Part model, mm, in its own coordinate system. A direction names the side the tool comes from. Round coordinates to 2 decimals unless told otherwise and drop trailing zeros. Order: outer loops, then holes, each group sorted by start corner. A loop starts at its lowest first (then second) coordinate and runs counter-clockwise, first axis right, second up. Notation, with made-up numbers: (34, -3) - (92, -3) arc R23 ccw to (92, 21) - close; hole circle Ø7 at (-28, 3). An arc over 180 degrees is marked (long way). Return JSON: item names as keys, results as strings. Group by question number.
Item 1: Saw through at A-A on y = 46.5. List the corners of the cut face in (x, z).
Item 2: Saw through at B-B on z = -22.5. List the corners of the cut face in (x, y).
Item 3: Tool access for faces 1 (the face through (1, 83, -68.5)), 2 (the face through (1, 81, -17)), 3 (the face through (2, 9, -24.5)): list every direction of +Z, -Z, +X, -X, +Y, -Y with a clear straight run to the whole face (end or side of a thin tool).
Item 4: Probe probe 1 along Z at (x, y) = (2.8, 35.5); probe 2 along Y at (x, z) = (1.6, -96.5); probe 3 along Z at (x, y) = (2.15, 7). List the from-to ranges inside material, lowest first.
Item 5: Saw through at D-D on x = 0.5. State how many separate pieces and enclosed holes the cut face has, and give its area (3 significant figures).
Item 6: Drop a flat-ended pin along its axis: pin 1 (2.5 mm diameter, centred on y = 6, z = -8.5, fed in from -X) (3 decimals). Give the stop position or say it passes through.
Item 7: Two-plate mould, pull along Z, no slides. Class faces 4 (the face through (1, 81, -88)), 5 (the face through (1, 40, -105)), 6 (the face through (2, 9, -80.5)): released by +Z, released by -Z, zero draft, split by the parting line, or undercut.
Item 8: Saw through at C-C on y = 6. List the corners of the cut face in (x, z), and give its area (3 significant figures).
```python
from build123d import *

# Parameters (mm, degrees)
CROQUIS1_R              = 1.5
CROQUIS1_W              = 3
CROQUIS1_H              = 32
SALIENTE_EXTRUIR1_DEPTH = 3
CORTAR_EXTRUIR1_DEPTH   = 3
CORTAR_EXTRUIR2_DEPTH   = 3


with BuildPart() as part:
    # Croquis1 → Saliente-Extruir1 (new body)
    with BuildSketch(Plane(origin=(0, 0, 0), x_dir=(0, 0, -1), z_dir=(1, 0, 0))):
        Polygon((0, 0), (105, 0), (105, 81), (84.5, 81), (84.5, 84), (68.5, 84), (68.5, 81), (36.5, 81), (36.5, 84), (20.5, 84), (20.5, 81), (0, 81), align=None)
        with Locations((8.5, 71)):
            Circle(CROQUIS1_R, mode=Mode.SUBTRACT)
        with Locations((96.5, 71)):
            Circle(CROQUIS1_R, mode=Mode.SUBTRACT)
        with Locations((8.5, 6)):
            Circle(CROQUIS1_R, mode=Mode.SUBTRACT)
        with Locations(Location((96.5, 6, 0), (0, 0, 180))):
            Circle(CROQUIS1_R, mode=Mode.SUBTRACT)
        with Locations((8.5, 33)):
            Rectangle(CROQUIS1_W, CROQUIS1_H, mode=Mode.SUBTRACT)
        with Locations((96.5, 33)):
            Rectangle(CROQUIS1_W, CROQUIS1_H, mode=Mode.SUBTRACT)
    extrude(amount=SALIENTE_EXTRUIR1_DEPTH)

    # Croquis2 → Cortar-Extruir1 (cut)
    with BuildSketch(Plane(origin=(3, 0, 0), x_dir=(0, 0, -1), z_dir=(1, 0, 0))):
        with BuildLine():
            Line((14, 79), (14, 81))
            Line((14, 81), (11, 81))
            Line((11, 81), (11, 79))
            Line((11, 79), (10.25, 79))
            ThreePointArc((10.25, 79), (9.823223305, 79.176776695), (10, 78.75))
            Line((10, 78.75), (10, 76.25))
            ThreePointArc((10, 76.25), (9.823223305, 75.823223305), (10.25, 76))
            Line((10.25, 76), (11, 76))
            Line((11, 76), (11, 75))
            Line((11, 75), (14, 75))
            Line((14, 75), (14, 76))
            Line((14, 76), (14.75, 76))
            ThreePointArc((14.75, 76), (15.176776695, 75.823223305), (15, 76.25))
            Line((15, 76.25), (15, 78.75))
            ThreePointArc((15, 78.75), (15.176776695, 79.176776695), (14.75, 79))
            Line((14.75, 79), (14, 79))
        make_face()
        with BuildLine():
            Line((94, 79), (94, 81))
            Line((94, 81), (91, 81))
            Line((91, 81), (91, 79))
            Line((91, 79), (90.25, 79))
            ThreePointArc((90.25, 79), (89.823223305, 79.176776695), (90, 78.75))
            Line((90, 78.75), (90, 76.25))
            ThreePointArc((90, 76.25), (89.823223305, 75.823223305), (90.25, 76))
            Line((90.25, 76), (91, 76))
            Line((91, 76), (91, 75))
            Line((91, 75), (94, 75))
            Line((94, 75), (94, 76))
            Line((94, 76), (94.75, 76))
            ThreePointArc((94.75, 76), (95.176776695, 75.823223305), (95, 76.25))
            Line((95, 76.25), (95, 78.75))
            ThreePointArc((95, 78.75), (95.176776695, 79.176776695), (94.75, 79))
            Line((94.75, 79), (94, 79))
        make_face()
    extrude(amount=-CORTAR_EXTRUIR1_DEPTH, mode=Mode.SUBTRACT)

    # Croquis3 → Cortar-Extruir2 (cut)
    with BuildSketch(Plane(origin=(3, 0, 0), x_dir=(0, 0, -1), z_dir=(1, 0, 0))):
        with BuildLine():
            Line((20.5, 4.122846639), (20.5, 13.122846639))
            ThreePointArc((20.5, 13.122846639), (22.5, 15.122846639), (24.5, 13.122846639))
            Line((24.5, 13.122846639), (24.5, 4.122846639))
            ThreePointArc((24.5, 4.122846639), (22.5, 2.122846639), (20.5, 4.122846639))
        make_face()
        with BuildLine():
            Line((84.5, 4.122846639), (84.5, 13.122846639))
            ThreePointArc((84.5, 13.122846639), (82.5, 15.122846639), (80.5, 13.122846639))
            Line((80.5, 13.122846639), (80.5, 4.122846639))
            ThreePointArc((80.5, 4.122846639), (82.5, 2.122846639), (84.5, 4.122846639))
        make_face()
    extrude(amount=-CORTAR_EXTRUIR2_DEPTH, mode=Mode.SUBTRACT)


solid = part.part
```
Filled in:
{
 "1": {"outline": "(0, -105) - (3, -105) - (3, -98) - (0, -98) - close; (0, -95) - (3, -95) - (3, -10) - (0, -10) - close; (0, -7) - (3, -7) - (3, 0) - (0, 0) - close"},
 "2": {"outline": "(0, 0) - (3, 0) - (3, 2.12) - (0, 2.12) - close; (0, 15.12) - (3, 15.12) - (3, 84) - (0, 84) - close"},
 "3": {"face 1": "+X, -X, +Y", "face 2": "+Z, +X, -X, +Y", "face 3": "+X, -X"},
 "4": {"probe 1": "z = -105 to -98, -95 to -10, -7 to 0", "probe 2": "y = 0 to 4.5, 7.5 to 17, 49 to 69.5, 72.5 to 81", "probe 3": "z = -105 to -97.62, -95.38 to -84.5, -80.5 to -24.5, -20.5 to -9.62, -7.38 to 0"},
 "5": {"separate pieces": "1", "enclosed holes": "8", "area": "8,230 mm^2"},
 "6": {"pin 1": "passes through"},
 "7": {"face 4": "zero draft", "face 5": "released by -Z", "face 6": "undercut"},
 "8": {"outline": "(0, -105) - (3, -105) - (3, -98) - (0, -98) - close; (0, -95) - (3, -95) - (3, -84.5) - (0, -84.5) - close; (0, -80.5) - (3, -80.5) - (3, -24.5) - (0, -24.5) - close; (0, -20.5) - (3, -20.5) - (3, -10) - (0, -10) - close; (0, -7) - (3, -7) - (3, 0) - (0, 0) - close", "area": "273 mm^2"}
}
